Geometry check sheet. Reference: the model listing, model coordinates, mm. Face numbers are marked on the shaded views. A direction names the side the tool comes from. Coordinates: 2 decimals unless noted, no trailing zeros. Loops run counter-clockwise (first coordinate to the right, second up) from the corner with the lowest first, then second, coordinate; pieces in that order, holes last.
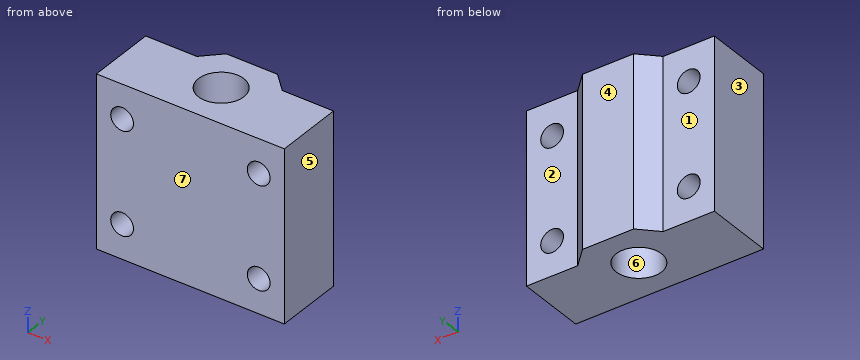
from build123d import *

# Parameters (mm, degrees)
ESQUISSE1_W             = 33
ESQUISSE1_H             = 30
BOSS_EXTRU_1_DEPTH      = 15
ESQUISSE2_R             = 4
ENL_V_MAT_EXTRU_1_DEPTH = 38.379807383
ENL_V_MAT_EXTRU_2_DEPTH = 38.379807383
ESQUISSE4_R             = 2
ENL_V_MAT_EXTRU_3_DEPTH = 26.322914524


with BuildPart() as part:
    # Esquisse1 → Boss.-Extru.1 (new body)
    with BuildSketch(Plane(origin=(0, 0, 0), x_dir=(1, 0, 0), z_dir=(0, 1, 0))):
        Rectangle(ESQUISSE1_W, ESQUISSE1_H)
    extrude(amount=BOSS_EXTRU_1_DEPTH)

    # Esquisse2 → Enlèv. mat.-Extru.1 (cut, through all)
    with BuildSketch(Plane.XY.offset(15)):
        with Locations((0, 7.5)):
            Circle(ESQUISSE2_R)
    extrude(amount=-ENL_V_MAT_EXTRU_1_DEPTH, mode=Mode.SUBTRACT)

    # Esquisse3 → Enlèv. mat.-Extru.2 (cut, through all)
    with BuildSketch(Plane.XY.offset(15)):
        Polygon((-16.5, 15), (-16.5, 12), (-7.5, 12), (-4.5, 15), align=None)
    enl_v_mat_extru_2 = extrude(amount=-ENL_V_MAT_EXTRU_2_DEPTH, mode=Mode.SUBTRACT)

    # Symétrie1: Enlèv. mat.-Extru.2 across plane
    add(enl_v_mat_extru_2.mirror(Plane(origin=(0, 0, 0), x_dir=(0, 0, 1), z_dir=(1, 0, 0))), mode=Mode.SUBTRACT)

    # Esquisse4 → Enlèv. mat.-Extru.3 (cut, through all)
    with BuildSketch(Plane(origin=(0, 12, 0), x_dir=(1, 0, 0), z_dir=(0, 1, 0))):
        with Locations(Location((-12, 9, 0), (0, 0, 270))):
            Circle(ESQUISSE4_R)
        with Locations(Location((12, 9, 0), (0, 0, 270))):
            Circle(ESQUISSE4_R)
        with Locations(Location((-12, -9, 0), (0, 0, 270))):
            Circle(ESQUISSE4_R)
        with Locations(Location((12, -9, 0), (0, 0, 270))):
            Circle(ESQUISSE4_R)
    extrude(amount=-ENL_V_MAT_EXTRU_3_DEPTH, mode=Mode.SUBTRACT)


solid = part.part
1) Access from +Z, -Z, +X, -X, +Y, -Y to the whole of each face (thin tool, end or side, straight path). Record for the marked faces 1, 2 and 3.
Data:
face 1: +Z, -Z, -X, +Y
face 2: +Z, -Z, +X, +Y
face 3: +Z, -Z, -X, +Y, -Y
2) Section check C-C on y = 7.5. Record the cut outline in (x, z).
Data:
outline: (-16.5, -15) - (-4, -15) - (-4, 15) - (-16.5, 15) - close; (4, -15) - (16.5, -15) - (16.5, 15) - (4, 15) - close; hole circle Ø4 at (-12, -9); hole circle Ø4 at (-12, 9); hole circle Ø4 at (12, -9); hole circle Ø4 at (12, 9)
3) Section check B-B on z = -9. Record the cut outline in (x, y).
Data:
outline: (-16.5, 0) - (-14, 0) - (-14, 12) - (-16.5, 12) - close; (-10, 0) - (10, 0) - (10, 12) - (7.5, 12) - (4.5, 15) - (-4.5, 15) - (-7.5, 12) - (-10, 12) - close; (14, 0) - (16.5, 0) - (16.5, 12) - (14, 12) - close; hole circle Ø8 at (0, 7.5)
4) Mould release check, pull along Y, two halves, no side actions. Record for the marked faces 4, 5, 6 and 7: +Y half, -Y half, draft (parallel to the pull), parting line (faces both ways), or undercut.
Data:
face 4: +Y half
face 5: draft
face 6: undercut
face 7: -Y half
5) Material ranges on probe 1 along Z at (x, y) = (13, 2.5); probe 2 along X at (y, z) = (8.25, -7.5); probe 3 along X at (y, z) = (2.5, -9), recorded low to high.
Data:
probe 1: z = -15 to -10.73, -7.27 to 7.27, 10.73 to 15
probe 2: x = -16.5 to -13.32, -10.68 to -3.93, 3.93 to 10.68, 13.32 to 16.5
probe 3: x = -16.5 to -14, -10 to 10, 14 to 16.5
6) Depth check by flat-ended pin: pin 1 (5 mm diameter, centred on x = 0, y = 7.5, fed in from -Z); pin 2 (10 mm diameter, centred on x = -13, z = 4, fed in from +Y). Enter the tip coordinate at first touch or a pass-through.
Data:
pin 1: passes through
pin 2: stops at y = 12
7) Section check D-D on x = 0. Record the cut outline in (y, z).
Data:
outline: (0, -15) - (3.5, -15) - (3.5, 15) - (0, 15) - close; (11.5, -15) - (15, -15) - (15, 15) - (11.5, 15) - close
8) Section check A-A on x = -12. Record the cut outline in (y, z).
Data:
outline: (0, -15) - (12, -15) - (12, -11) - (0, -11) - close; (0, -7) - (12, -7) - (12, 7) - (0, 7) - close; (0, 11) - (12, 11) - (12, 15) - (0, 15) - close
